```python
from build123d import *

# Parameters (mm, degrees)
SKETCH1_R               = 4
BOSS_EXTRUDE1_DEPTH     = 2
SKETCH2_R               = 2.75
BOSS_EXTRUDE2_DEPTH     = 12.6
SKETCH3_R               = 3.9
BOSS_EXTRUDE3_DEPTH     = 1.5
SKETCH4_R               = 2
BOSS_EXTRUDE4_DEPTH     = 6
FILLET1_R               = 1
BOSS_EXTRUDE5_DEPTH     = 3.6
SKETCH6_R               = 0.5
BOSS_EXTRUDE6_DEPTH     = 57
CUT_EXTRUDE1_DEPTH      = 5
CUT_EXTRUDE1_DEPTH_BACK = 5
FILLET2_R               = 0.4


with BuildPart() as part:
    # Sketch1 → Boss-Extrude1 (new body)
    with BuildSketch(Plane.XY):
        Circle(SKETCH1_R)
    extrude(amount=BOSS_EXTRUDE1_DEPTH)

    # Sketch2 → Boss-Extrude2 (add)
    with BuildSketch(Plane.XY.offset(2)):
        Circle(SKETCH2_R)
    extrude(amount=BOSS_EXTRUDE2_DEPTH)

    # Sketch3 → Boss-Extrude3 (add)
    with BuildSketch(Plane.XY.offset(14.6)):
        Circle(SKETCH3_R)
    extrude(amount=BOSS_EXTRUDE3_DEPTH)

    # Sketch4 → Boss-Extrude4 (add)
    with BuildSketch(Plane.XY.offset(16.1)):
        Circle(SKETCH4_R)
    extrude(amount=BOSS_EXTRUDE4_DEPTH)

    # Fillet1
    fillet1_edges = [part.edges().sort_by_distance(p)[0] for p in [
        (-2, 0, 22.1),
    ]]
    fillet(fillet1_edges, radius=FILLET1_R)

    # Sketch5 → Boss-Extrude5 (add)
    with BuildSketch(Plane(origin=(0, 0, 0), x_dir=(1, 0, 0), z_dir=(0, 1, 0))):
        Polygon((-0.5, -5), (0.5, -5), (0.5, -10.6), (1, -10.6), (0, -12.8), (-1, -10.6), (-0.5, -10.6), align=None)
    extrude(amount=BOSS_EXTRUDE5_DEPTH)

    # Sketch6 → Boss-Extrude6 (add)
    with BuildSketch(Plane.XY.offset(22.1)):
        Circle(SKETCH6_R)
    extrude(amount=BOSS_EXTRUDE6_DEPTH)

    # Sketch7 → Cut-Extrude1 (cut, two sides)
    with BuildSketch(Plane(origin=(0, 0, 0), x_dir=(0, 0, -1), z_dir=(1, 0, 0))) as cut_extrude1_sk:
        Polygon((-79.1, 0.5), (-77.1, -0.5), (-79.1, -0.5), align=None)
    extrude(amount=CUT_EXTRUDE1_DEPTH, mode=Mode.SUBTRACT)
    extrude(cut_extrude1_sk.sketch, amount=-CUT_EXTRUDE1_DEPTH_BACK, mode=Mode.SUBTRACT)

    # Fillet2
    fillet2_edges = [part.edges().sort_by_distance(p)[0] for p in [
        (-3.9, 0, 14.6),
        (-3.9, 0, 16.1),
    ]]
    fillet(fillet2_edges, radius=FILLET2_R)


solid = part.part
```
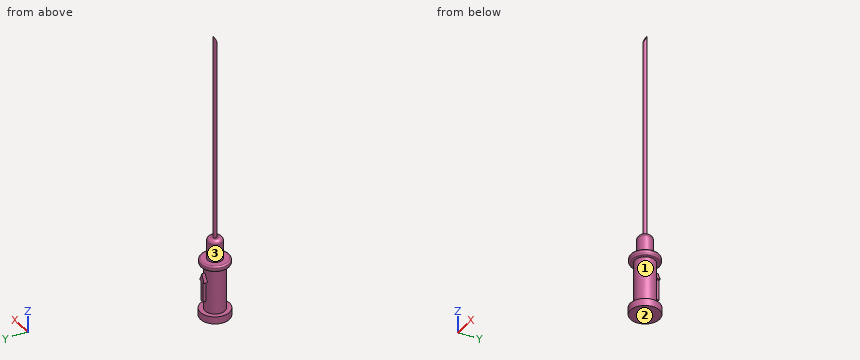
Check sheet for the modelled part. Datum: model origin and axes. Units: mm. Face numbers are marked on the shaded views. Give positions to 0.01 mm unless a question says otherwise; leave off trailing zeros. Order: outer loops, then holes, each group sorted by start corner. A loop starts at its lowest first (then second) coordinate and runs counter-clockwise, first axis right, second up. Notation, with made-up numbers: M 57,79 L 86,79 A11 ccw 86,97 Z; hole C 47,-25.5 d7. An arc over 180 degrees is marked long. Answer in a Markdown table with one row per item.
1) Release check for a two-part mould opening along Z. For the marked faces 1, 2 and 3 record: +Z half, -Z half, draft (parallel to the pull), parting line (faces both ways), or undercut.
Filled sheet:
| item | result |
|---|---|
| face 1 | undercut |
| face 2 | -Z half |
| face 3 | draft |
2) Gauge pin test, flat ends, axial feed: P1, Ø1, axis at x = 0, y = -0.5, coming from the +Z side; P2, Ø1.5, axis at x = 0, y = 0, coming from the +Z side; P3, Ø1, axis at x = 0.5, z = 10.5, coming from the +Y side; P4, Ø0.7, axis at y = 3.5, z = 7, coming from the +X side. Record the tip position at first contact, or that the pin passes through.
Filled sheet:
| item | result |
|---|---|
| P1 | stops at z = 78.1 |
| P2 | stops at z = 79.1 |
| P3 | stops at y = 3.6 |
| P4 | stops at x = 0.5 |
3) Cross-section at A-A, the plane z = 55.5. Enter the section's corners in (x, y).
Filled sheet:
| item | result |
|---|---|
| outline | C 0,0 d1 |
4) Thickness scan on L1, parallel to Z at x = -3, y = 0.5; L2, parallel to Z at x = 0.25, y = -2.25; L3, parallel to Z at x = -1, y = -0.5. Record the ranges inside material, lowest first. Write a range as [from, to].
Filled sheet:
| item | result |
|---|---|
| L1 | z = [0, 2], [14.6, 16.1] |
| L2 | z = [0, 16.1] |
| L3 | z = [0, 22.09] |
